Read the model definition and answer for the solid it produces. Units are mm, in the model's axes. Face numbers are marked on the shaded views. Give positions to 0.01 mm unless a question says otherwise; leave off trailing zeros. Write each loop counter-clockwise with the first axis right and the second up, starting at its lowest first coordinate (ties: lowest second). Pieces come first, ordered by that corner, then holes. Notation, with made-up numbers: M 87,-12.5 L 104,-12.5 A34 cw 104,22.5 Z; hole C -34.5,66 d10. An arc over 180 degrees is marked long. Use a Markdown table: item, result. Add a question column.
Item 1: A cutting plane is placed at C-C on x = -7. Determine the outline of the cut face in (y, z) (3 decimals), then the cut area to 3 significant figures.
Item 2: A cutting plane is placed at D-D on z = 2.9. Determine the outline of the cut face in (x, y).
Item 3: Consider probe 1 along Y at (x, z) = (0, 5.2); probe 2 along Y at (x, z) = (0, 3.8); probe 3 along Y at (x, z) = (2.5, 1.1). Determine where each line is inside the solid, lowest interval first. Write a range as [from, to].
Item 4: The mould has two halves that part along Y. Classify the marked faces 1, 2 and 3: pulls with the +Y half, pulls with the -Y half, needs draft (parallel to the pull), parting line crosses it, or undercut.
Item 5: Given P1, Ø3, axis at y = 0.5, z = 1, coming from the -X side; P2, Ø1.9, axis at x = -15, y = 0, coming from the -Z side; P3, Ø2, axis at y = -10, z = 1, coming from the +X side, each flat-ended and moving along its own axis, determine where each tip first touches the part or whether it passes through.
Item 6: A cutting plane is placed at A-A on y = 0. Determine the outline of the cut face in (x, z), then the cut area to 3 significant figures.
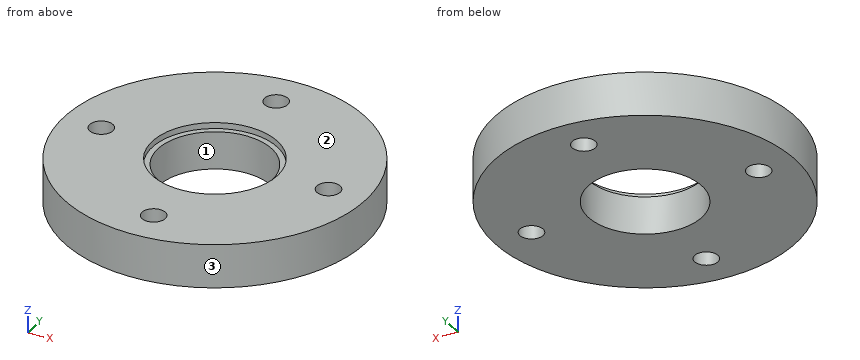
from build123d import *

# Parameters (mm, degrees)
SKETCH_1_R          = 20
SKETCH_1_R_2        = 7.55
SKETCH_1_R_3        = 1.55
EXTRUDE_1_DEPTH     = 5.8
SKETCH_2_R          = 8.3
CUT_EXTRUDE_1_DEPTH = 0.8


with BuildPart() as part:
    # ｽｹｯﾁ1 → ﾎﾞｽ - 押し出し1 (new body)
    with BuildSketch(Plane.XY):
        Circle(SKETCH_1_R)
        Circle(SKETCH_1_R_2, mode=Mode.SUBTRACT)
        with Locations((0, 15)):
            Circle(SKETCH_1_R_3, mode=Mode.SUBTRACT)
        with Locations((15, 0)):
            Circle(SKETCH_1_R_3, mode=Mode.SUBTRACT)
        with Locations((0, -15)):
            Circle(SKETCH_1_R_3, mode=Mode.SUBTRACT)
        with Locations((-15, 0)):
            Circle(SKETCH_1_R_3, mode=Mode.SUBTRACT)
    extrude(amount=EXTRUDE_1_DEPTH)

    # ｽｹｯﾁ2 → ｶｯﾄ - 押し出し1 (cut)
    with BuildSketch(Plane.XY.offset(5.8)):
        Circle(SKETCH_2_R)
    extrude(amount=-CUT_EXTRUDE_1_DEPTH, mode=Mode.SUBTRACT)


solid = part.part
Filled in:
| question | item | result |
|---|---|---|
| 1 | outline | M -18.735,0 L -2.829,0 L -2.829,5 L -4.46,5 L -4.46,5.8 L -18.735,5.8 Z; M 2.829,0 L 18.735,0 L 18.735,5.8 L 4.46,5.8 L 4.46,5 L 2.829,5 Z |
| 1 | area | 182 mm² |
| 2 | outline | C 0,0 d40; hole C -15,0 d3.1; hole C 0,0 d15.1; hole C 0,-15 d3.1; hole C 0,15 d3.1; hole C 15,0 d3.1 |
| 3 | probe 1 | [-20, -16.55], [-13.45, -8.3], [8.3, 13.45], [16.55, 20] |
| 3 | probe 2 | [-20, -16.55], [-13.45, -7.55], [7.55, 13.45], [16.55, 20] |
| 3 | probe 3 | [-19.84, -7.12], [7.12, 19.84] |
| 4 | face 1 | undercut |
| 4 | face 2 | needs draft |
| 4 | face 3 | parting line crosses it |
| 5 | P1 | x = -20 |
| 5 | P2 | through |
| 5 | P3 | x = 17.86 |
| 6 | outline | M -20,0 L -16.55,0 L -16.55,5.8 L -20,5.8 Z; M -13.45,0 L -7.55,0 L -7.55,5 L -8.3,5 L -8.3,5.8 L -13.45,5.8 Z; M 7.55,0 L 13.45,0 L 13.45,5.8 L 8.3,5.8 L 8.3,5 L 7.55,5 Z; M 16.55,0 L 20,0 L 20,5.8 L 16.55,5.8 Z |
| 6 | area | 107 mm² |
